from build123d import *


with BuildPart() as part:
    # Sketch2 → Revolve1 (revolve)
    with BuildSketch(Plane.ZY.offset(-259.301545348)):
        Polygon((0, -133.573704322), (5, -133.573704322), (5, -131.573704322), (47.330517131, -131.573704322), (47.330517131, -128.573704322), (5, -128.573704322), (5, -119.573704322), (52.330517131, -119.573704322), (52.330517131, -114.573704322), (0, -114.573704322), align=None)
    revolve(axis=Axis((259.301545348, -148.573704322, -1.12), (0, 0, 1)))


solid = part.part
Model file for the job. Use its own axes, mm. A direction names the side the tool comes from. Give positions to 0.01 mm unless a question says otherwise; leave off trailing zeros. Loops run counter-clockwise (first coordinate to the right, second up) from the corner with the lowest first, then second, coordinate; pieces in that order, holes last.
1) Tool access for faces 4 (the flat face through (271, -159, 5)), 5 (the flat face through (274, -141, 0)): list every direction of +Z, -Z, +X, -X, +Y, -Y with a clear straight run to the whole face (end or side of a thin tool).
2) Saw through at B-B (y = -149). Write the cut outline in (x, z).
3) Flat gauge pins, fed straight in: pin 1 Ø1.5 at (y, z) = (-123.5, 23) entering from +X; pin 2 Ø3 at (y, z) = (-157.5, 18) entering from -X; pin 3 Ø3 at (y, z) = (-138, 11) entering from +X. Where does each tip first touch, or does it go through?
4) Saw through at C-C (z = 12.5). Write the cut outline in (x, y).
5) Saw through at D-D (y = -121). Write the cut outline in (x, z), plus the area to 3 significant figures.
6) Saw through at A-A (x = 273). Write the cut outline in (y, z), plus the area to 3 significant figures.
7) Wall check: line 1 (X direction, y = -133, z = 31.5); line 2 (X direction, y = -146.5, z = 10.5); line 3 (Y direction, x = 258, z = 12.5). Give the ranges that are in metal, low to high.
8) Pull direction Y, two halves, no side cores. Call faces 1 (the cylindrical face through (272.324, -117.166, 25.799)), 2 (the cylindrical face through (276.948, -171.587, 28.997)), 3 (the flat face through (244, -174, 52.331)): +Y half, -Y half, draft (parallel to the pull), parting line (faces both ways), or undercut.
Answer block:
1. face 4: +Z
1. face 5: -Z, +X, -X, +Y, -Y
2. outline: (225.3, 0) - (244.31, 0) - (244.31, 5) - (242.31, 5) - (242.31, 47.33) - (239.31, 47.33) - (239.31, 5) - (230.3, 5) - (230.3, 52.33) - (225.3, 52.33) - close; (274.3, 0) - (293.3, 0) - (293.3, 52.33) - (288.3, 52.33) - (288.3, 5) - (279.3, 5) - (279.3, 47.33) - (276.3, 47.33) - (276.3, 5) - (274.3, 5) - close
3. pin 1: stops at x = 283.06
3. pin 2: stops at x = 226.12
3. pin 3: stops at x = 292.07
4. outline: circle Ø68 at (259.3, -148.57); circle Ø40 at (259.3, -148.57); hole circle Ø58 at (259.3, -148.57); hole circle Ø34 at (259.3, -148.57)
5. outline: (239.41, 0) - (279.19, 0) - (279.19, 52.33) - (268.28, 52.33) - (268.28, 5) - (250.32, 5) - (250.32, 52.33) - (239.41, 52.33) - close
5. area: 1,230 mm2
6. outline: (-179.69, 0) - (-154.69, 0) - (-154.69, 5) - (-158.64, 5) - (-158.64, 47.33) - (-163.15, 47.33) - (-163.15, 5) - (-174.13, 5) - (-174.13, 52.33) - (-179.69, 52.33) - close; (-142.46, 0) - (-117.46, 0) - (-117.46, 52.33) - (-123.01, 52.33) - (-123.01, 5) - (-134, 5) - (-134, 47.33) - (-138.51, 47.33) - (-138.51, 5) - (-142.46, 5) - close
6. area: 1,160 mm2
7. line 1: x = 229.08 to 234.84, 246.75 to 252.49, 266.12 to 271.85, 283.76 to 289.53
7. line 2: x = 225.36 to 230.38, 239.41 to 242.43, 276.17 to 279.19, 288.23 to 293.24
7. line 3: y = -182.55 to -177.54, -168.53 to -165.52, -131.62 to -128.62, -119.6 to -114.6
8. face 1: parting line
8. face 2: undercut
8. face 3: draft
